Autodesk Inventor part; units mm, degrees
ref_plane "YZ Plane" through (0, 0, 0) normal (1, 0, 0) x (0, 1, 0)
ref_plane "XZ Plane" through (0, 0, 0) normal (0, 1, 0) x (-1, 0, 0)
ref_plane "XY Plane" through (0, 0, 0) normal (0, 0, 1) x (1, 0, 0)
sketch "草圖1" plane through (0, 0, 0) normal (0, 0, 1) x (1, 0, 0)
  circle A0 centre (0, 0) radius 5
  line L0 (0, 0) -> (0, 100) construction
  line L1 (12.5, 0) -> (12.5, 100)
  line L2 (-12.5, 100) -> (-12.5, 0)
  arc A1 (-12.5, 0) -> (12.5, 0) centre (0, 0) ccw
  arc A2 (12.5, 100) -> (-12.5, 100) centre (0, 100) ccw
  point P0 (0, 50)
  dimension "d0" = 10
  dimension "d1" = 100
  dimension "d2" = 25
extrude "擠出1" add sketch "草圖1" along normal blind 3
Design review of the part built by this model. Coordinates are the model's own, in mm. Round coordinates to 2 decimals unless told otherwise and drop trailing zeros. Order: outer loops, then holes, each group sorted by start corner. A loop starts at its lowest first (then second) coordinate and runs counter-clockwise, first axis right, second up. Notation, with made-up numbers: (-27, -18.5) - (0, -18.5) arc R34 ccw to (0, 17.5) - close; hole circle Ø4 at (64, 84.25). An arc over 180 degrees is marked (long way). Return JSON: item names as keys, results as strings.
Q1. The part is to be moulded in two halves that separate along Y. For faces 1 (the cylindrical face through (-1.08, 4.88, 1.48)), 2 (the flat face through (-12.5, 51, 1)), 3 (the cylindrical face through (0.275, -12.497, 1.479)), 4 (the cylindrical face through (-0.275, 112.497, 1.479)), say which applies: pulls with the +Y half, pulls with the -Y half, needs draft (parallel to the pull), parting line crosses it, or undercut.
Computed values:
{"face 1": "undercut", "face 2": "needs draft", "face 3": "pulls with the -Y half", "face 4": "pulls with the +Y half"}
Q2. Consider section C-C on x = -8. Write out the cut boundary in (y, z), plus the area to 3 significant figures.
Computed values:
{"outline": "(-9.6, 0) - (109.6, 0) - (109.6, 3) - (-9.6, 3) - close", "area": "358 mm2"}
Q3. For pin 1 Ø1 at (x, z) = (-9, 1.5) entering from -Y, flat-tipped, find the tip position at first contact; note if it passes through.
Computed values:
{"pin 1": "stops at y = -9.17"}
Q4. Consider section A-A on x = 0. Write out the cut boundary in (y, z), plus the area to 3 significant figures.
Computed values:
{"outline": "(-12.5, 0) - (-5, 0) - (-5, 3) - (-12.5, 3) - close; (5, 0) - (112.5, 0) - (112.5, 3) - (5, 3) - close", "area": "345 mm2"}
Q5. Wall thickness on L1, parallel to Y at x = 0, z = 2; L2, parallel to Y at x = 4.5, z = 0.25; L3, parallel to Y at x = -9, z = 0.95: over which ranges is each line inside the solid? List them lowest first. Write a range as [from, to].
Computed values:
{"L1": "y = [-12.5, -5], [5, 112.5]", "L2": "y = [-11.66, -2.18], [2.18, 111.66]", "L3": "y = [-8.67, 108.67]"}
Q6. Consider section B-B on z = 2.4. Write out the cut boundary in (x, y), plus the area to 3 significant figures.
Computed values:
{"outline": "(-12.5, 0) arc R12.5 ccw to (12.5, 0) - (12.5, 100) arc R12.5 ccw to (-12.5, 100) - close; hole circle Ø10 at (0, 0)", "area": "2,910 mm2"}
